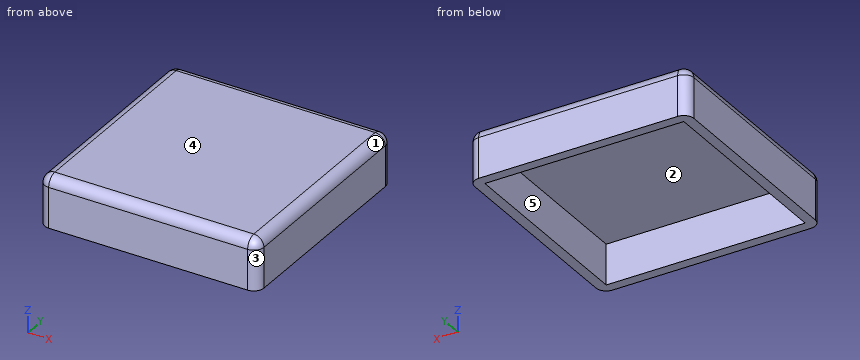
```python
from build123d import *

# Parameters (mm, degrees)
F0_W     = 65
F0_H     = 65
F1_DEPTH = 15
F2_R     = 3
F3_T     = 3


# Not quite as in the source:
# - a shell that OpenCascade refuses in one call is made with other operations: the cavity is built on its own and cut out


with BuildPart() as f1:
    # F0 (on Top) → F1 (new body)
    with BuildSketch(Plane.XY):
        Rectangle(F0_W, F0_H)
    extrude(amount=F1_DEPTH)

    # F2
    f2_edges = [f1.edges().sort_by_distance(p)[0] for p in [
        (0, -32.5, 15),
        (32.5, 0, 15),
        (0, 32.5, 15),
        (-32.5, 0, 15),
        (-32.5, 32.5, 7.5),
        (-32.5, -32.5, 7.5),
        (32.5, 32.5, 7.5),
        (32.5, -32.5, 7.5),
    ]]
    fillet(f2_edges, radius=F2_R)

    # F3: shell of thickness 3, made by hand


with BuildPart() as f3_core1:
    # F3_t2: copy of F1
    add(f1.part)

    # the walls: a layer under each face that stays
    f3_faces = [f3_core1.faces().sort_by_distance(p)[0] for p in [
        (0, -32.5, 6),
        (-32.5, 0, 6),
        (32.5, 0, 6),
        (0, 32.5, 6),
        (0, 0, 15),
    ]]
    thicken(f3_faces, amount=-F3_T, mode=Mode.SUBTRACT)


with BuildPart() as f1_1:
    add(f1.part)

    # what is left inside the walls is the cavity
    f3_cavity = [f3_core1.part.solids().sort_by_distance(p)[0] for p in [
        (0, -9.833333, 0.03),
    ]]
    add(f3_cavity, mode=Mode.SUBTRACT)


solid = f1_1.part
```
Read the model definition and answer for the solid it produces. Units are mm, in the model's axes. Face numbers are marked on the shaded views. A direction names the side the tool comes from. Coordinates: 2 decimals unless noted, no trailing zeros. Write each loop counter-clockwise with the first axis right and the second up, starting at its lowest first coordinate (ties: lowest second). Pieces come first, ordered by that corner, then holes. Notation, with made-up numbers: (41.5, 39.5) - (63.5, 39.5) arc R16 cw to (63.5, 66.5) - close; hole circle Ø9 at (-24, 58). An arc over 180 degrees is marked (long way). Answer as a JSON object with one key per item and string values. Group by question number.
1. Consider L1, parallel to Y at x = -10, z = 11; L2, parallel to Z at x = 12, y = 3. Determine where each line is inside the solid, lowest interval first. Write a range as [from, to].
2. A cutting plane is placed at A-A (z = 5.5). Determine the outline of the cut face in (x, y), plus the area to 3 significant figures.
3. Which of the six approach directions +Z, -Z, +X, -X, +Y, -Y give full straight-line access (tool end or side, diameter ignored) to the marked faces 1 and 2?
4. The mould has two halves that part along X. Classify the marked faces 3, 4 and 5: +X half, -X half, draft (parallel to the pull), parting line (faces both ways), or undercut.
5. A cutting plane is placed at B-B (x = -8.5). Determine the outline of the cut face in (y, z), plus the area to 3 significant figures.
6. A cutting plane is placed at D-D (z = 14.25). Determine the outline of the cut face in (x, y), plus the area to 3 significant figures.
7. This flat-tipped pin is pushed along its axis until it touches: P1, Ø17.5, axis at x = 10.5, y = 0, coming from the -Z side. Where does it stop, or does it pass through?
Worked out:
{
 "1": {"L1": "y = [-32.5, -29.5], [29.5, 32.5]", "L2": "z = [12, 15]"},
 "2": {"outline": "(-32.5, -29.5) arc R3 ccw to (-29.5, -32.5) - (29.5, -32.5) arc R3 ccw to (32.5, -29.5) - (32.5, 29.5) arc R3 ccw to (29.5, 32.5) - (-29.5, 32.5) arc R3 ccw to (-32.5, 29.5) - close; hole (-29.5, -29.5) - (29.5, -29.5) - (29.5, 29.5) - (-29.5, 29.5) - close", "area": "736 mm²"},
 "3": {"face 1": "+Z, +X, +Y, -Y", "face 2": "-Z"},
 "4": {"face 3": "+X half", "face 4": "draft", "face 5": "undercut"},
 "5": {"outline": "(-32.5, 0) - (-29.5, 0) - (-29.5, 12) - (29.5, 12) - (29.5, 0) - (32.5, 0) - (32.5, 12) arc R3 ccw to (29.5, 15) - (-29.5, 15) arc R3 ccw to (-32.5, 12) - close", "area": "263 mm²"},
 "6": {"outline": "(-31.48, -29.5) arc R1.98 ccw to (-29.5, -31.48) - (29.5, -31.48) arc R1.98 ccw to (31.48, -29.5) - (31.48, 29.5) arc R1.98 ccw to (29.5, 31.48) - (-29.5, 31.48) arc R1.98 ccw to (-31.48, 29.5) - close", "area": "3,960 mm²"},
 "7": {"P1": "stops at z = 12"}
}
